Job drawing, mm, ordinate dimensions from the low corner. One solid piece. A direction names the side the tool comes from. Give positions to 0.01 mm unless a question says otherwise; leave off trailing zeros. Order: outer loops, then holes, each group sorted by start corner. A loop starts at its lowest first (then second) coordinate and runs counter-clockwise, first axis right, second up.
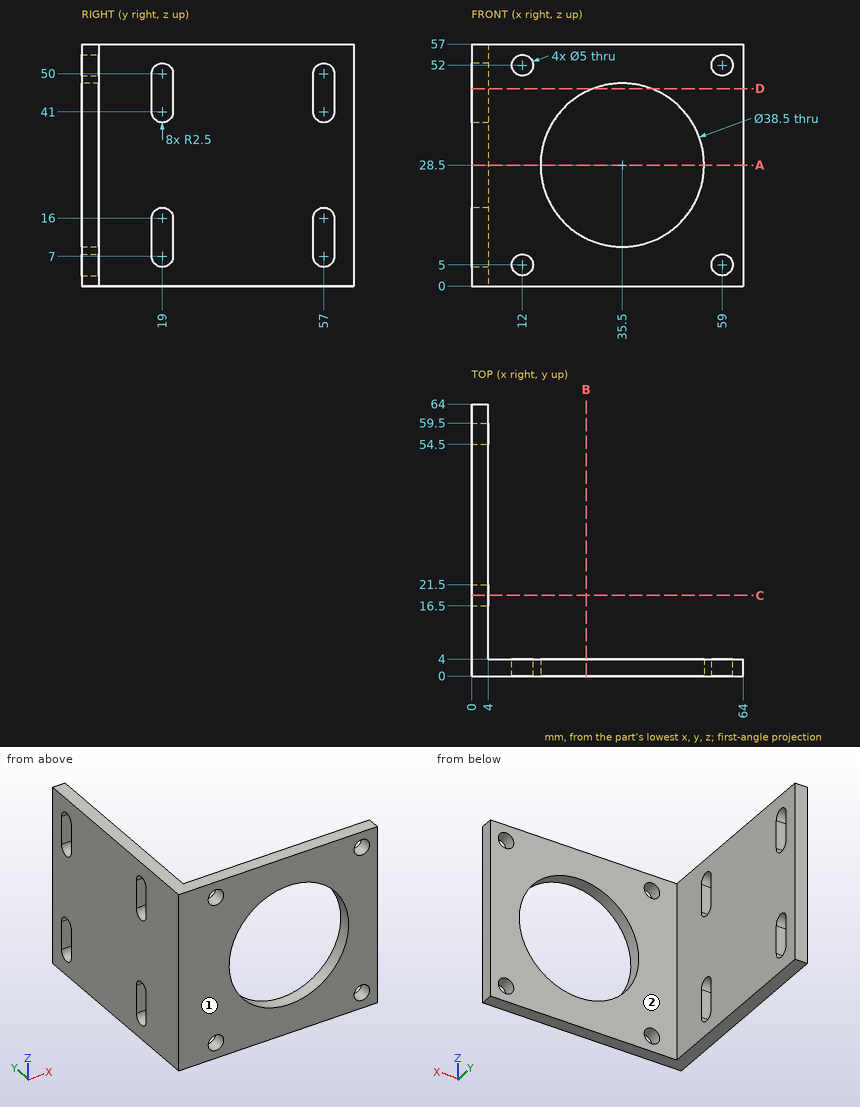
Item 1: Drill centre lines: probe 1 along Z at (x, y) = (12, 1); probe 2 along X at (y, z) = (1.35, 5); probe 3 along Z at (x, y) = (35, 1). Where is each one in solid material? Low to high.
Item 2: Band-saw the part on D-D on z = 46.5. List the corners of the cut face in (x, y), plus the area to 3 significant figures.
Item 3: Drop flat-ended pins along their axis: P1, Ø2, axis at x = 16, z = 38, coming from the +Y side; P2, Ø3, axis at y = 53, z = 50, coming from the +X side; P3, Ø23, axis at x = 35.5, z = 28.5, coming from the +Y side. Give the stop position or say it passes through.
Item 4: Band-saw the part on A-A on z = 28.5. List the corners of the cut face in (x, y).
Item 5: Band-saw the part on C-C on y = 19. List the corners of the cut face in (x, z).
Item 6: Which spindle directions (+Z, -Z, +X, -X, +Y, -Y) get a long thin tool onto all of the face, cutting with end or side? Do the marked faces 1 and 2. Say none if no direction does.
Item 7: Band-saw the part on B-B on x = 27. List the corners of the cut face in (y, z), plus the area to 3 significant figures.
Working result:
1. probe 1: z = 0 to 2.5, 7.5 to 49.5, 54.5 to 57
1. probe 2: x = 0 to 9.5, 14.5 to 56.5, 61.5 to 64
1. probe 3: z = 0 to 9.26, 47.74 to 57
2. outline: (0, 0) - (28.68, 0) - (28.68, 4) - (4, 4) - (4, 16.5) - (0, 16.5) - close; (0, 21.5) - (4, 21.5) - (4, 54.5) - (0, 54.5) - close; (0, 59.5) - (4, 59.5) - (4, 64) - (0, 64) - close; (42.32, 0) - (64, 0) - (64, 4) - (42.32, 4) - close
2. area: 401 mm2
3. P1: stops at y = 4
3. P2: stops at x = 4
3. P3: passes through
4. outline: (0, 0) - (16.25, 0) - (16.25, 4) - (4, 4) - (4, 64) - (0, 64) - close; (54.75, 0) - (64, 0) - (64, 4) - (54.75, 4) - close
5. outline: (0, 0) - (4, 0) - (4, 4.5) - (0, 4.5) - close; (0, 18.5) - (4, 18.5) - (4, 38.5) - (0, 38.5) - close; (0, 52.5) - (4, 52.5) - (4, 57) - (0, 57) - close
6. face 1: +Z, -Z, +X, -X, -Y
6. face 2: +Z, -Z, +X, +Y
7. outline: (0, 0) - (4, 0) - (4, 11.23) - (0, 11.23) - close; (0, 45.77) - (4, 45.77) - (4, 57) - (0, 57) - close
7. area: 89.8 mm2
